Can you work these out from the drawing? Everything is in mm from the part's minimum corner. A direction names the side the tool comes from. Coordinates: 2 decimals unless noted, no trailing zeros. Loops run counter-clockwise (first coordinate to the right, second up) from the corner with the lowest first, then second, coordinate; pieces in that order, holes last.
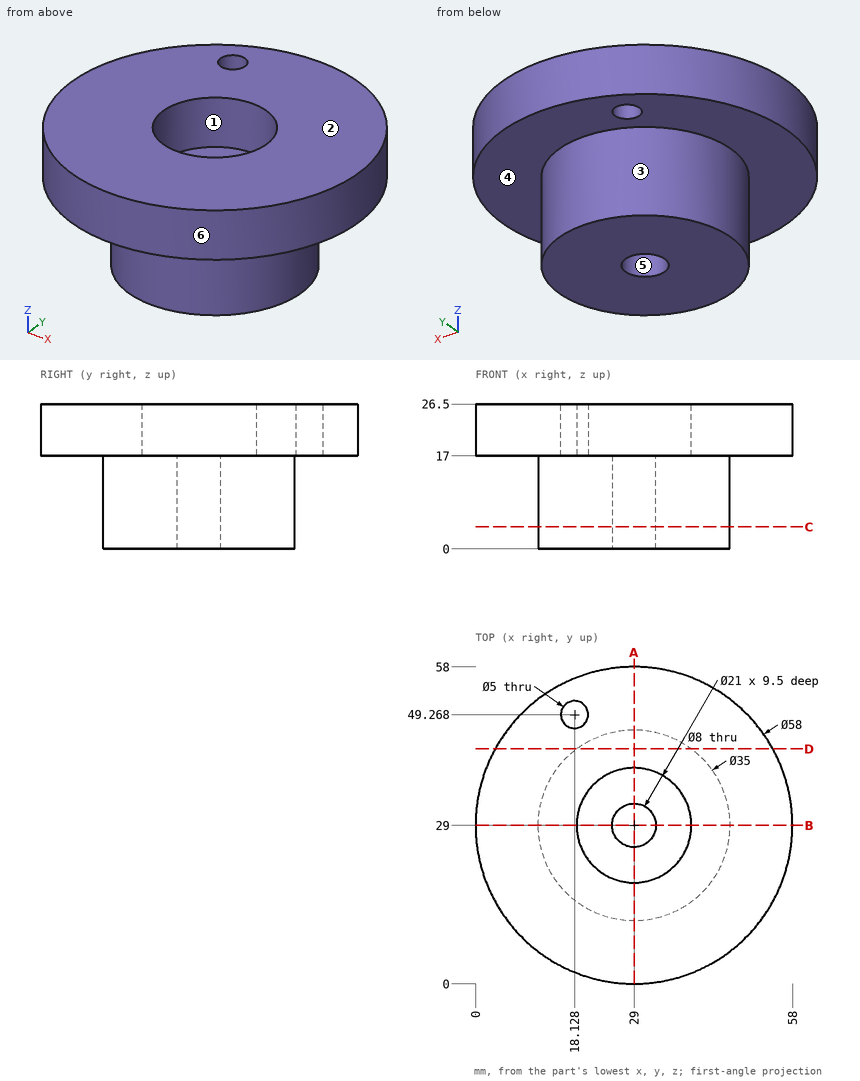
Item 1: I need wall thicknesses on line 1 along Y through (x, z) = (29, 10.25); line 2 along Z through (x, y) = (49, 15); line 3 along Z through (x, y) = (22.5, 23). Which ranges of each line are inside material? Lowest first, please.
Results are:
line 1: y = 11.5 to 25, 33 to 46.5
line 2: z = 17 to 26.5
line 3: z = 0 to 17
Item 2: Suppose I cut it at A-A, the plane x = 29. Please give me the cut outline in (y, z).
Results are:
outline: (0, 17) - (11.5, 17) - (11.5, 0) - (25, 0) - (25, 17) - (18.5, 17) - (18.5, 26.5) - (0, 26.5) - close; (33, 0) - (46.5, 0) - (46.5, 17) - (58, 17) - (58, 26.5) - (39.5, 26.5) - (39.5, 17) - (33, 17) - close
Item 3: Suppose I cut it at C-C, the plane z = 4. Please give me the cut outline in (x, y), plus the area to 3 significant figures.
Results are:
outline: circle Ø35 at (29, 29); hole circle Ø8 at (29, 29)
area: 912 mm2
Item 4: We'd pull the mould along Y, two halves only. Please class the marked faces 4, 5 and 6: +Y half, -Y half, draft (parallel to the pull), parting line (faces both ways), or undercut.
Results are:
face 4: draft
face 5: undercut
face 6: parting line
Item 5: I'm going to push flat-ended pins straight in: P1, Ø10.5, axis at x = 32.5, y = 30, coming from the +Z side; P2, Ø10, axis at y = 41, z = 20, coming from the -X side; P3, Ø3, axis at y = 20.5, z = 7.5, coming from the +X side; P4, Ø4, axis at x = 18.13, y = 49.27, coming from the +Z side. Where does each tip first touch, or does it pass through?
Results are:
P1: stops at z = 17
P2: stops at x = 0.86
P3: stops at x = 45.04
P4: passes through
Item 6: Suppose I cut it at D-D, the plane y = 43. Please give me the cut outline in (x, z).
Results are:
outline: (3.6, 17) - (18.5, 17) - (18.5, 0) - (39.5, 0) - (39.5, 17) - (54.4, 17) - (54.4, 26.5) - (3.6, 26.5) - close
Item 7: On a 3-axis mill with a long thin cutter (end or side, diameter ignored), from which of +Z, -Z, +X, -X, +Y, -Y can I reach the whole of each face in a straight line? I mean the marked faces 1, 2 and 3. Say none if no direction works.
Results are:
face 1: +Z
face 2: +Z, +X, -X, +Y, -Y
face 3: -Z
